Source: CAD feature listing. Evaluate the final solid. Frame: model axes, mm. Round coordinates to 2 decimals unless told otherwise and drop trailing zeros. Loops run counter-clockwise (first coordinate to the right, second up) from the corner with the lowest first, then second, coordinate; pieces in that order, holes last. Notation, with made-up numbers: (14.5, 36.5) - (49.5, 36.5) arc R14 ccw to (49.5, 49.5) - close; hole circle Ø2 at (11.25, -10). An arc over 180 degrees is marked (long way). One line per question, with ' | ' between items. Start each with the question number.
1. Cut plane B-B (z = 19.05). Return loops of the section in (x, y), then the cut area to 3 significant figures.
2. Cut plane A-A (x = 19.05). Return loops of the section in (y, z).
3. Mould query, pull axis Z, two halves, no side actions, for faces 1 (the cylindrical face through (67.32, 18.78, 18.72)), 2 (the flat face through (44, 19, 38.1)), 3 (the flat face through (0, 19, 19)), 4 (the flat face through (44, 19, 0)). Classes: pulls with the +Z half, pulls with the -Z half, needs draft (parallel to the pull), parting line crosses it, or undercut.
4. Ray query, line 1 (X direction, y = 24.5, z = 19.05); line 2 (Z direction, x = 19, y = 29); line 3 (X direction, y = 27.5, z = 20.5). Return the intervals inside material, ascending.
Autodesk Inventor part; units mm, degrees
ref_plane "YZ Plane" through (0, 0, 0) normal (1, 0, 0) x (0, 1, 0)
ref_plane "XZ Plane" through (0, 0, 0) normal (0, 1, 0) x (-1, 0, 0)
ref_plane "XY Plane" through (0, 0, 0) normal (0, 0, 1) x (1, 0, 0)
sketch "Sketch1" plane through (0, 0, 0) normal (0, 0, 1) x (1, 0, 0)
  line L0 (0, 0) -> (88.9, 0)
  line L1 (88.9, 0) -> (88.9, 38.1)
  line L2 (88.9, 38.1) -> (0, 38.1)
  line L3 (0, 38.1) -> (0, 0)
  dimension "d0" = 88.9
  dimension "d1" = 38.1
extrude "Extrusion1" add sketch "Sketch1" along normal blind 38.1
sketch "Sketch2" plane through (0, 38.1, 0) normal (0, 1, 0) x (1, 0, 0)
  line L0 (88.9, 0) -> (0, 0)
  line L1 (0, 0) -> (0, -38.1)
  line L2 (88.9, -38.1) -> (0, -38.1)
  circle A0 centre (19.05, -19.05) radius 5.8141
  circle A1 centre (69.85, -19.05) radius 5.8141
  dimension "d4" = 19.05
  dimension "d5" = 19.05
  dimension "d8" = 50.8
hole "Hole1" at (19.05, 38.1, 19.05) at (69.85, 38.1, 19.05) direction (0, -1, 0) diameter 5.1054 end through all
equation "\"d18\" = d8"
properties part number "hubjig_spacer" material "Wood (Cherry)"
Answers follow:
1) outline: (0, 0) - (16.5, 0) - (16.5, 38.1) - (0, 38.1) - close; (21.6, 0) - (67.3, 0) - (67.3, 38.1) - (21.6, 38.1) - close; (72.4, 0) - (88.9, 0) - (88.9, 38.1) - (72.4, 38.1) - close | area: 3,000 mm2
2) outline: (0, 0) - (38.1, 0) - (38.1, 16.5) - (0, 16.5) - close; (0, 21.6) - (38.1, 21.6) - (38.1, 38.1) - (0, 38.1) - close
3) face 1: undercut | face 2: pulls with the +Z half | face 3: needs draft | face 4: pulls with the -Z half
4) line 1: x = 0 to 16.5, 21.6 to 67.3, 72.4 to 88.9 | line 2: z = 0 to 16.5, 21.6 to 38.1 | line 3: x = 0 to 16.95, 21.15 to 67.75, 71.95 to 88.9
